```python
from build123d import *

# Parameters (mm, degrees)
SKETCH1_W                       = 355.6
SKETCH1_H                       = 203.2
BASE_FLANGE1_DEPTH              = 3.2639
EDGE_FLANGE1_STRIP_W            = 18.36928
EDGE_FLANGE1_STRIP_H            = 3.2639
EDGE_FLANGE1_STRIP_CUT_DEPTH    = 203.2
EDGE_FLANGE1_DEPTH              = 203.2
EDGE_FLANGE2_DEPTH              = 241.3
CUT_EXTRUDE1_DEPTH              = 450.37928505
EDGE_FLANGE3_DEPTH              = 177.8
EDGE_FLANGE3_BEND_DEPTH         = 177.8
FILLET1_R                       = 3.175
F_1_4_START                     = -177.8
F_1_4_0_25_DIAMETER_SLOT1_DEPTH = 355.6
F_1_4_START_2                   = -3.2639
F_1_4_0_25_DIAMETER_SLOT2_DEPTH = 3.2639
F_1_4_0_25_DIAMETER_SLOT3_DEPTH = 3.2639


# Read off the part's stored shape, not the designer's step: 1/4 (0.25) Diameter Slot1, 1/4 (0.25) Diameter Slot2, 1/4 (0.25) Diameter Slot3
# Sheet-metal steps are written as plain solids
with BuildPart() as part:
    # Sketch1 → Base-Flange1 (new body)
    with BuildSketch(Plane(origin=(0, 0, 0), x_dir=(1, 0, 0), z_dir=(0, 1, 0))):
        Rectangle(SKETCH1_W, SKETCH1_H)
    extrude(amount=-BASE_FLANGE1_DEPTH)

    # Edge-Flange1 strip (across the edge) → Edge-Flange1 strip cut (cut)
    with BuildSketch(Plane(origin=(177.8, 0, 101.6), x_dir=(-1, 0, 0), z_dir=(0, 0, -1))):
        with Locations((-3.2639, -1.63195)):
            Rectangle(EDGE_FLANGE1_STRIP_W, EDGE_FLANGE1_STRIP_H)
    edge_flange1_strip_cut = extrude(amount=EDGE_FLANGE1_STRIP_CUT_DEPTH, mode=Mode.SUBTRACT)

    # Edge-Flange1 section (across the edge) → Edge-Flange1 (add)
    with BuildSketch(Plane(origin=(177.8, 0, 101.6), x_dir=(-1, 0, 0), z_dir=(0, 0, -1))):
        with BuildLine():
            Line((0, 2.65684), (0, 250.7361))
            Line((0, 250.7361), (3.2639, 250.7361))
            Line((3.2639, 250.7361), (3.2639, 2.65684))
            ThreePointArc((3.2639, 2.65684), (4.042070419, 0.778170419), (5.92074, 0))
            Line((5.92074, 0), (5.92074, -3.2639))
            ThreePointArc((5.92074, -3.2639), (1.734144596, -1.529755404), (0, 2.65684))
        make_face()
    edge_flange1 = extrude(amount=EDGE_FLANGE1_DEPTH)

    # Edge-Flange2 section (across the edge) → Edge-Flange2 (add)
    with BuildSketch(Plane(origin=(174.5361, 250.7361, -109.08284), x_dir=(0, 0, 1), z_dir=(0, -1, 0))):
        with BuildLine():
            Line((-3.2639, 2.65684), (-3.2639, 34.8361))
            Line((-3.2639, 34.8361), (0, 34.8361))
            Line((0, 34.8361), (0, 2.65684))
            ThreePointArc((0, 2.65684), (0.778170419, 0.778170419), (2.65684, 0))
            Line((2.65684, 0), (7.48284, 0))
            Line((7.48284, 0), (7.48284, -3.2639))
            Line((7.48284, -3.2639), (2.65684, -3.2639))
            ThreePointArc((2.65684, -3.2639), (-1.529755404, -1.529755404), (-3.2639, 2.65684))
        make_face()
    edge_flange2 = extrude(amount=EDGE_FLANGE2_DEPTH)

    # Sketch14 → Cut-Extrude1 (cut, through all)
    with BuildSketch(Plane(origin=(177.8, 0, 0), x_dir=(0, 0, -1), z_dir=(1, 0, 0))):
        with BuildLine():
            Line((74.24674, 250.7361), (74.24674, 60.2361))
            ThreePointArc((74.24674, 60.2361), (66.807252242, 42.275587758), (48.84674, 34.8361))
            Line((48.84674, 34.8361), (-76.2, 34.8361))
            ThreePointArc((-76.2, 34.8361), (-94.160512242, 27.396612242), (-101.6, 9.4361))
            Line((-101.6, 9.4361), (-101.6, 250.7361))
            Line((-101.6, 250.7361), (74.24674, 250.7361))
        make_face()
    cut_extrude1 = extrude(amount=-CUT_EXTRUDE1_DEPTH, mode=Mode.SUBTRACT)

    # Mirror1: Edge-Flange1 strip cut, Edge-Flange1, Edge-Flange2, Cut-Extrude1 across plane
    add(edge_flange1_strip_cut.mirror(Plane(origin=(0, 0, 0), x_dir=(0, 0, 1), z_dir=(1, 0, 0))), mode=Mode.SUBTRACT)
    add(edge_flange1.mirror(Plane(origin=(0, 0, 0), x_dir=(0, 0, 1), z_dir=(1, 0, 0))))
    add(edge_flange2.mirror(Plane(origin=(0, 0, 0), x_dir=(0, 0, 1), z_dir=(1, 0, 0))))
    add(cut_extrude1.mirror(Plane(origin=(0, 0, 0), x_dir=(0, 0, 1), z_dir=(1, 0, 0))), mode=Mode.SUBTRACT)

    # Edge-Flange3 section (across the edge) → Edge-Flange3 (add)
    with BuildSketch(Plane(origin=(174.5361, 72.9361, -65.2399), x_dir=(0, 0, -1), z_dir=(0, 1, 0))):
        with BuildLine():
            Line((-3.2639, 2.65684), (-3.2639, 22.1361))
            Line((-3.2639, 22.1361), (0, 22.1361))
            Line((0, 22.1361), (0, 2.65684))
            ThreePointArc((0, 2.65684), (0.778170419, 0.778170419), (2.65684, 0))
            Line((2.65684, 0), (9.00684, 0))
            Line((9.00684, 0), (9.00684, -3.2639))
            Line((9.00684, -3.2639), (2.65684, -3.2639))
            ThreePointArc((2.65684, -3.2639), (-1.529755404, -1.529755404), (-3.2639, 2.65684))
        make_face()
    extrude(amount=EDGE_FLANGE3_DEPTH)

    # Edge-Flange3 section 2 (across the edge) → Edge-Flange3 bend (add)
    with BuildSketch(Plane(origin=(-174.5361, 250.7361, -65.2399), x_dir=(0, 0, -1), z_dir=(0, -1, 0))):
        with BuildLine():
            Line((-3.2639, 2.65684), (-3.2639, 22.1361))
            Line((-3.2639, 22.1361), (0, 22.1361))
            Line((0, 22.1361), (0, 2.65684))
            ThreePointArc((0, 2.65684), (0.778170419, 0.778170419), (2.65684, 0))
            Line((2.65684, 0), (9.00684, 0))
            Line((9.00684, 0), (9.00684, -3.2639))
            Line((9.00684, -3.2639), (2.65684, -3.2639))
            ThreePointArc((2.65684, -3.2639), (-1.529755404, -1.529755404), (-3.2639, 2.65684))
        make_face()
    extrude(amount=EDGE_FLANGE3_BEND_DEPTH)

    # Fillet1
    fillet1_edges = [part.edges().sort_by_distance(p)[0] for p in [
        (-176.16805, 9.4361, -101.6),
        (-139.7, 9.4361, -110.71479),
        (-139.7, 250.7361, -110.71479),
        (176.16805, 72.9361, -74.24674),
        (-176.16805, 72.9361, -74.24674),
        (176.16805, 9.4361, -101.6),
        (139.7, 250.7361, -110.71479),
        (139.7, 9.4361, -110.71479),
    ]]
    fillet(fillet1_edges, radius=FILLET1_R)

    # 1/4 (0.25) Diameter Slot1 outline → 1/4 (0.25) Diameter Slot1 (cut)
    with BuildSketch(Plane.YZ.offset(F_1_4_START)):
        with BuildLine():
            Line((79.2861, -99.64674), (91.9861, -99.64674))
            ThreePointArc((91.9861, -99.64674), (95.1611, -96.47174), (91.9861, -93.29674))
            Line((91.9861, -93.29674), (79.2861, -93.29674))
            ThreePointArc((79.2861, -93.29674), (76.1111, -96.47174), (79.2861, -99.64674))
        make_face()
        with BuildLine():
            ThreePointArc((231.6861, -99.64674), (234.8611, -96.47174), (231.6861, -93.29674))
            Line((231.6861, -93.29674), (218.9861, -93.29674))
            ThreePointArc((218.9861, -93.29674), (215.8111, -96.47174), (218.9861, -99.64674))
            Line((218.9861, -99.64674), (231.6861, -99.64674))
        make_face()
    extrude(amount=F_1_4_0_25_DIAMETER_SLOT1_DEPTH, mode=Mode.SUBTRACT)

    # 1/4 (0.25) Diameter Slot2 outline → 1/4 (0.25) Diameter Slot2 (cut)
    with BuildSketch(Plane(origin=(0, 0, 0), x_dir=(1, 0, 0), z_dir=(0, 1, 0)).offset(F_1_4_START_2)):
        with BuildLine():
            ThreePointArc((95.25, -3.175), (98.425, -6.35), (101.6, -3.175))
            Line((101.6, -3.175), (101.6, 9.525))
            ThreePointArc((101.6, 9.525), (98.425, 12.7), (95.25, 9.525))
            Line((95.25, 9.525), (95.25, -3.175))
        make_face()
        with BuildLine():
            ThreePointArc((101.6, -69.85), (98.425, -66.675), (95.25, -69.85))
            Line((95.25, -69.85), (95.25, -82.55))
            ThreePointArc((95.25, -82.55), (98.425, -85.725), (101.6, -82.55))
            Line((101.6, -82.55), (101.6, -69.85))
        make_face()
        with BuildLine():
            ThreePointArc((158.75, -69.85), (155.575, -66.675), (152.4, -69.85))
            Line((152.4, -69.85), (152.4, -82.55))
            ThreePointArc((152.4, -82.55), (155.575, -85.725), (158.75, -82.55))
            Line((158.75, -82.55), (158.75, -69.85))
        make_face()
        with BuildLine():
            ThreePointArc((158.75, 9.525), (155.575, 12.7), (152.4, 9.525))
            Line((152.4, 9.525), (152.4, -3.175))
            ThreePointArc((152.4, -3.175), (155.575, -6.35), (158.75, -3.175))
            Line((158.75, -3.175), (158.75, 9.525))
        make_face()
    f_1_4_0_25_diameter_slot2 = extrude(amount=F_1_4_0_25_DIAMETER_SLOT2_DEPTH, mode=Mode.SUBTRACT)

    # Mirror2: 1/4 (0.25) Diameter Slot2 across plane
    add(f_1_4_0_25_diameter_slot2.mirror(Plane(origin=(0, 0, 0), x_dir=(0, 0, 1), z_dir=(1, 0, 0))), mode=Mode.SUBTRACT)

    # 1/4 (0.25) Diameter Slot3 outline → 1/4 (0.25) Diameter Slot3 (cut)
    with BuildSketch(Plane(origin=(0, 0, 0), x_dir=(1, 0, 0), z_dir=(0, 1, 0)).offset(F_1_4_START_2)):
        with BuildLine():
            ThreePointArc((-44.45, 61.54674), (-47.625, 58.37174), (-44.45, 55.19674))
            Line((-44.45, 55.19674), (-31.75, 55.19674))
            ThreePointArc((-31.75, 55.19674), (-28.575, 58.37174), (-31.75, 61.54674))
            Line((-31.75, 61.54674), (-44.45, 61.54674))
        make_face()
        with BuildLine():
            ThreePointArc((44.45, 55.19674), (47.625, 58.37174), (44.45, 61.54674))
            Line((44.45, 61.54674), (31.75, 61.54674))
            ThreePointArc((31.75, 61.54674), (28.575, 58.37174), (31.75, 55.19674))
            Line((31.75, 55.19674), (44.45, 55.19674))
        make_face()
    extrude(amount=F_1_4_0_25_DIAMETER_SLOT3_DEPTH, mode=Mode.SUBTRACT)


solid = part.part
```
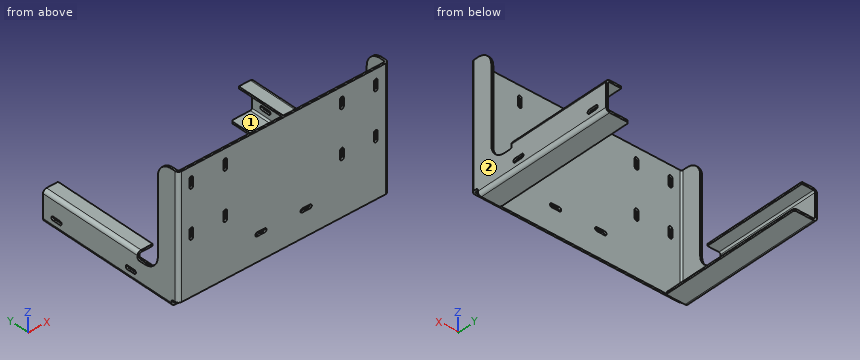
Geometry check sheet. Reference: the model listing, model coordinates, mm. Face numbers are marked on the shaded views. A direction names the side the tool comes from. Give positions to 0.01 mm unless a question says otherwise; leave off trailing zeros. Write each loop counter-clockwise with the first axis right and the second up, starting at its lowest first coordinate (ties: lowest second). Pieces come first, ordered by that corner, then holes.
1) Section check B-B, the plane x = 40. Record the boundary of the cut face in (y, z), and give its area (4 significant figures).
2) Section check A-A, the plane y = 83.5. State how many separate pieces and enclosed holes the cut face has, and give its area (3 significant figures).
3) Gauge pin test, flat ends, axial feed: pin 1 (6 mm diameter, centred on x = -80, z = -62.5, fed in from +Y); pin 2 (3.5 mm diameter, centred on x = -38.5, y = -2, fed in from -Z); pin 3 (2.5 mm diameter, centred on x = 176, y = 226, fed in from +Z). Record the tip position at first contact, or that the pin passes through.
4) Section check C-C, the plane y = 160. Record the boundary of the cut face in (x, z), and give its area (3 significant figures).
5) Material ranges on L1, parallel to Z at x = 158, y = 82; L2, parallel to X at y = 84.5, z = -80.5; L3, parallel to Y at x = 94.5, z = 21, recorded low to high.
6) Access from +Z, -Z, +X, -X, +Y, -Y to the whole of each face (thin tool, end or side, straight path). Record for the marked faces 1 and 2.
7) Section check D-D, the plane z = 51. Record the boundary of the cut face in (x, y).
Computed:
1. outline: (-3.26, -101.6) - (0, -101.6) - (0, -61.55) - (-3.26, -61.55) - close; (-3.26, -55.2) - (0, -55.2) - (0, 101.6) - (-3.26, 101.6) - close
1. area: 642.5 mm2
2. separate pieces: 4
2. enclosed holes: 0
2. area: 635 mm2
3. pin 1: stops at y = 0
3. pin 2: stops at z = -101.6
3. pin 3: stops at z = -62.72
4. outline: (-177.8, -106.43) arc R5.92 ccw to (-171.88, -112.35) - (-139.7, -112.35) - (-139.7, -109.08) - (-171.88, -109.08) arc R2.66 cw to (-174.54, -106.43) - (-174.54, -67.9) arc R2.66 cw to (-171.88, -65.24) - (-152.4, -65.24) - (-152.4, -61.98) - (-171.88, -61.98) arc R5.92 ccw to (-177.8, -67.9) - close; (139.7, -112.35) - (171.88, -112.35) arc R5.92 ccw to (177.8, -106.43) - (177.8, -67.9) arc R5.92 ccw to (171.88, -61.98) - (152.4, -61.98) - (152.4, -65.24) - (171.88, -65.24) arc R2.66 cw to (174.54, -67.9) - (174.54, -106.43) arc R2.66 cw to (171.88, -109.08) - (139.7, -109.08) - close
4. area: 677 mm2
5. L1: z = -112.35 to -109.08, -65.24 to -61.98
5. L2: x = -177.8 to -174.54, 174.54 to 177.8
5. L3: y = -3.26 to 0
6. face 1: +Y, -Y
6. face 2: +Z, -Z, +X, +Y, -Y
7. outline: (-177.8, 2.66) arc R5.92 ccw to (-171.88, -3.26) - (171.88, -3.26) arc R5.92 ccw to (177.8, 2.66) - (177.8, 34.84) - (174.54, 34.84) - (174.54, 2.66) arc R2.66 cw to (171.88, 0) - (-171.88, 0) arc R2.66 cw to (-174.54, 2.66) - (-174.54, 34.84) - (-177.8, 34.84) - close
